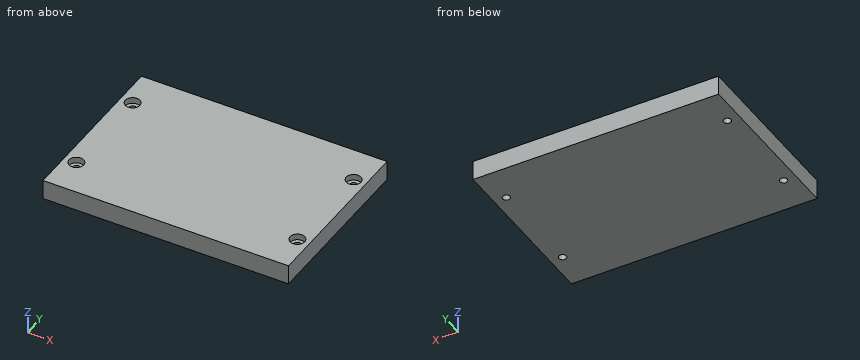
from build123d import *

# Parameters (mm, degrees)
SKETCH_W     = 200
SKETCH_H     = 140
SKETCH_R     = 3
PAD_DEPTH    = 16
SKETCH001_R  = 6
POCKET_DEPTH = 5


with BuildPart() as part:
    # Sketch → Pad (new body)
    with BuildSketch(Plane.XY):
        with Locations((100, 70)):
            Rectangle(SKETCH_W, SKETCH_H)
        with Locations((10, 110)):
            Circle(SKETCH_R, mode=Mode.SUBTRACT)
        with Locations((10, 30)):
            Circle(SKETCH_R, mode=Mode.SUBTRACT)
        with Locations((190, 110)):
            Circle(SKETCH_R, mode=Mode.SUBTRACT)
        with Locations((190, 30)):
            Circle(SKETCH_R, mode=Mode.SUBTRACT)
    extrude(amount=PAD_DEPTH)

    # Sketch001 (on Face10 of Pad) → Pocket (cut)
    with BuildSketch(Plane.XY.offset(16)):
        with Locations((10, 110)):
            Circle(SKETCH001_R)
        with Locations((190, 110)):
            Circle(SKETCH001_R)
        with Locations((190, 30)):
            Circle(SKETCH001_R)
        with Locations((10, 30)):
            Circle(SKETCH001_R)
    extrude(amount=-POCKET_DEPTH, mode=Mode.SUBTRACT)


solid = part.part
Could you check a few things on this model? Use its own coordinates, in mm. Give positions to 0.01 mm unless a question says otherwise; leave off trailing zeros. Order: outer loops, then holes, each group sorted by start corner. A loop starts at its lowest first (then second) coordinate and runs counter-clockwise, first axis right, second up.
1. Will this pin go through, and if not, where does the flat tip stop? P1, Ø6, axis at x = 11, y = 27.5, coming from the +Z side.
2. I need wall thicknesses on L1, parallel to Y at x = 10, z = 14.95; L2, parallel to Y at x = 190, z = 3.25. Which ranges of each line are inside material? Lowest first, please.
3. Suppose I cut it at B-B (x = 190). List the corners of the cut face in (y, z) for me.
4. Suppose I cut it at A-A (y = 110). List the corners of the cut face in (x, z) for me, plus the area to 3 significant figures.
Solved:
1. P1: stops at z = 11
2. L1: y = 0 to 24, 36 to 104, 116 to 140
2. L2: y = 0 to 27, 33 to 107, 113 to 140
3. outline: (0, 0) - (27, 0) - (27, 11) - (24, 11) - (24, 16) - (0, 16) - close; (33, 0) - (107, 0) - (107, 11) - (104, 11) - (104, 16) - (36, 16) - (36, 11) - (33, 11) - close; (113, 0) - (140, 0) - (140, 16) - (116, 16) - (116, 11) - (113, 11) - close
4. outline: (0, 0) - (7, 0) - (7, 11) - (4, 11) - (4, 16) - (0, 16) - close; (13, 0) - (187, 0) - (187, 11) - (184, 11) - (184, 16) - (16, 16) - (16, 11) - (13, 11) - close; (193, 0) - (200, 0) - (200, 16) - (196, 16) - (196, 11) - (193, 11) - close
4. area: 2,950 mm2
